For this review, take the finished solid that the model builds, in its own axes (mm). A direction names the side the tool comes from. Coordinates: 2 decimals unless noted, no trailing zeros. Write each loop counter-clockwise with the first axis right and the second up, starting at its lowest first coordinate (ties: lowest second). Pieces come first, ordered by that corner, then holes. Notation, with made-up numbers: (20.5, -26) -> (56.5, -26) arc R24 ccw to (56.5, -9) -> close; hole circle Ø11 at (-3, 60). An arc over 180 degrees is marked (long way). Put each result on its own line as item: value. Start each with the question number.
Item 1: For faces 1 (the flat face through (1, 1, 5.1)), 2 (the flat face through (1, 1, 0)), 3 (the flat face through (0, 0, -5)), list the 3-axis set-ups (+Z, -Z, +X, -X, +Y, -Y) from which the entire face can be reached by the end or side of a thin tool; tool diameter is ignored.
Item 2: Consider section D-D on y = -2.1. Give the boundary of the cut face in (x, z).
Item 3: To check wall thickness, follow L1, parallel to Z at x = 2.2, y = 0.8; L2, parallel to Y at x = -0.05, z = 5.75; L3, parallel to X at y = -1.2, z = 2.75. State the ranges of each line that lie inside material, in increasing order.
Item 4: Consider section A-A on x = 0.5. Give the boundary of the cut face in (y, z), and give its area (3 significant figures).
Item 5: Consider section B-B on y = 0.8. Give the boundary of the cut face in (x, z).
Item 6: Consider section C-C on z = 0.5. Give the boundary of the cut face in (x, y).
Autodesk Inventor part; units mm, degrees
ref_plane "YZ Plane" through (0, 0, 0) normal (1, 0, 0) x (0, 1, 0)
ref_plane "XZ Plane" through (0, 0, 0) normal (0, 1, 0) x (-1, 0, 0)
ref_plane "XY Plane" through (0, 0, 0) normal (0, 0, 1) x (1, 0, 0)
sketch "Sketch1" plane through (0, 0, 0) normal (0, 0, 1) x (1, 0, 0)
  circle A0 centre (0, 0) radius 1.2
  circle A1 centre (0, 0) radius 2.75
  line L0 (-1.75, 2.75) -> (1.75, 2.75)
  line L1 (2.75, 1.75) -> (2.75, -1.75)
  line L2 (1.75, -2.75) -> (-1.75, -2.75)
  line L3 (-2.75, -1.75) -> (-2.75, 1.75)
  arc A2 (-1.75, 2.75) -> (-2.75, 1.75) centre (-1.75, 1.75) ccw
  arc A3 (2.75, 1.75) -> (1.75, 2.75) centre (1.75, 1.75) ccw
  arc A4 (1.75, -2.75) -> (2.75, -1.75) centre (1.75, -1.75) ccw
  arc A5 (-2.75, -1.75) -> (-1.75, -2.75) centre (-1.75, -1.75) ccw
  point P0 (-2.75, 0)
  point P1 (0, -2.75)
  dimension "d0" = 2.4
  dimension "d1" = 5.5
  dimension "d2" = 1
  dimension "d3" = 1
  dimension "d4" = 1
extrude "Extrusion1" add sketch "Sketch1" against normal blind 5 contours A0
extrude "Extrusion2" add sketch "Sketch1" along normal blind 5.1 contours A0 | A1 | L1 A4 L2 A1 | A1 L0 A3 L1 | A1 L3 A2 L0
extrude "Extrusion3" add sketch "Sketch1" along normal blind 7.1 contours A0
properties part number "rpi_base_back_3DPrint"
Return value:
1. face 1: +Z
1. face 2: -Z
1. face 3: -Z, +X, -X, +Y, -Y
2. outline: (-1.78, 0) -> (2.69, 0) -> (2.69, 5.1) -> (-1.78, 5.1) -> close
3. L1: 0 to 5.1
3. L2: -1.2 to 1.2
3. L3: -2.47 to 2.75
4. outline: (-2.75, 0) -> (-1.09, 0) -> (-1.09, -5) -> (1.09, -5) -> (1.09, 0) -> (2.75, 0) -> (2.75, 5.1) -> (1.09, 5.1) -> (1.09, 7.1) -> (-1.09, 7.1) -> (-1.09, 5.1) -> (-2.75, 5.1) -> close
4. area: 43.3 mm^2
5. outline: (-2.75, 0) -> (-0.89, 0) -> (-0.89, -5) -> (0.89, -5) -> (0.89, 0) -> (2.75, 0) -> (2.75, 5.1) -> (0.89, 5.1) -> (0.89, 7.1) -> (-0.89, 7.1) -> (-0.89, 5.1) -> (-2.75, 5.1) -> close
6. outline: (-2.75, 0) arc R2.75 ccw to (0, -2.75) -> (1.75, -2.75) arc R1 ccw to (2.75, -1.75) -> (2.75, 1.75) arc R1 ccw to (1.75, 2.75) -> (-1.75, 2.75) arc R1 ccw to (-2.75, 1.75) -> close
